Autodesk Inventor part; units mm, degrees
ref_plane "YZ Plane" through (0, 0, 0) normal (1, 0, 0) x (0, 1, 0)
ref_plane "XZ Plane" through (0, 0, 0) normal (0, 1, 0) x (-1, 0, 0)
ref_plane "XY Plane" through (0, 0, 0) normal (0, 0, 1) x (1, 0, 0)
sketch "スケッチ1" plane through (0, 0, 0) normal (0, 1, 0) x (-1, 0, 0)
  line L0 (19, -14) -> (-19, -14)
  line L1 (-19, -14) -> (-19, 14)
  line L2 (-19, 14) -> (19, 14)
  line L3 (19, 14) -> (19, -14)
  line L4 (0, -27.2114) -> (0, 0) construction
  line L5 (0, 0) -> (-35.5982, 0) construction
  dimension "d0" = 28
  dimension "d1" = 38
extrude "押し出し1" add sketch "スケッチ1" along normal blind 2
sketch "スケッチ2" plane through (0, 2, 0) normal (0, 1, 0) x (1, 0, 0)
  circle A0 centre (0, 0) radius 11.5
  circle A1 centre (-16, 0) radius 1.7
  circle A2 centre (16, 0) radius 1.7
  line L0 (-19, 14) -> (-19, -14)
  line L1 (19, -14) -> (19, 14)
  dimension "d4" = 23
  dimension "d5" = 3.4
  dimension "d6" = 3.4
  dimension "d7" = 3
  dimension "d8" = 3
extrude "押し出し2" cut sketch "スケッチ2" against normal through all
properties part number "HayashiProbeHead_up" material "ステンレス鋼 440C"
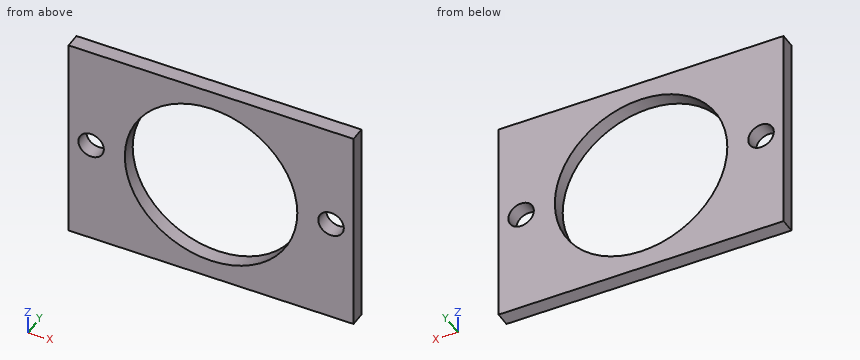
Part model, mm, in its own coordinate system. Round coordinates to 2 decimals unless told otherwise and drop trailing zeros. Write each loop counter-clockwise with the first axis right and the second up, starting at its lowest first coordinate (ties: lowest second). Pieces come first, ordered by that corner, then holes. Notation, with made-up numbers: M 89.25,33.5 L 103.25,33.5 A19 ccw 103.25,58.5 Z; hole C 46.5,70 d4. An arc over 180 degrees is marked long. One line per question, with ' | ' between items.
(1) Probe line 1 along X through (y, z) = (0.75, 0); line 2 along Z through (x, y) = (16, 1.55); line 3 along Z through (x, y) = (2, 0.45). List the from-to ranges inside material, lowest first.
Answer key:
line 1: x = -19 to -17.7, -14.3 to -11.5, 11.5 to 14.3, 17.7 to 19 | line 2: z = -14 to -1.7, 1.7 to 14 | line 3: z = -14 to -11.32, 11.32 to 14
(2) Saw through at D-D on z = 8.25. Write the cut outline in (x, y), then the cut area to 3 significant figures.
Answer key:
outline: M -19,0 L -8.01,0 L -8.01,2 L -19,2 Z; M 8.01,0 L 19,0 L 19,2 L 8.01,2 Z | area: 44.0 mm^2
(3) Pin check, flat tips, straight feed: pin 1 (4.5 mm diameter, centred on x = -16, z = 0, fed in from +Y); pin 2 (14 mm diameter, centred on x = 0, z = 0, fed in from -Y). Stop position of each tip, or through.
Answer key:
pin 1: stops at y = 2 | pin 2: passes through
(4) Saw through at B-B on y = 1. Write the cut outline in (x, z), then the cut area to 3 significant figures.
Answer key:
outline: M -19,-14 L 19,-14 L 19,14 L -19,14 Z; hole C -16,0 d3.4; hole C 0,0 d23; hole C 16,0 d3.4 | area: 630 mm^2
(5) Saw through at A-A on z = 0. Write the cut outline in (x, y).
Answer key:
outline: M -19,0 L -17.7,0 L -17.7,2 L -19,2 Z; M -14.3,0 L -11.5,0 L -11.5,2 L -14.3,2 Z; M 11.5,0 L 14.3,0 L 14.3,2 L 11.5,2 Z; M 17.7,0 L 19,0 L 19,2 L 17.7,2 Z
(6) Saw through at C-C on x = 0.5. Write the cut outline in (y, z).
Answer key:
outline: M 0,-14 L 2,-14 L 2,-11.49 L 0,-11.49 Z; M 0,11.49 L 2,11.49 L 2,14 L 0,14 Z
